Design review of the part built by this model. Coordinates are the model's own, in mm. Face numbers are marked on the shaded views. A direction names the side the tool comes from. Round coordinates to 2 decimals unless told otherwise and drop trailing zeros. Loops run counter-clockwise (first coordinate to the right, second up) from the corner with the lowest first, then second, coordinate; pieces in that order, holes last. Notation, with made-up numbers: (58, 52.25) -> (76, 52.25) arc R23 ccw to (76, 77.25) -> close; hole circle Ø2 at (37, 14). An arc over 180 degrees is marked (long way). Answer as CSV lines item,"result". Start each with the question number.
(1) For P1, Ø5, axis at y = -30.5, z = -21.5, coming from the -X side; P2, Ø13.5, axis at x = 10.37, z = 11.81, coming from the +Y side; P3, Ø15.5, axis at y = -61.5, z = -8.5, coming from the +X side; P4, Ø5, axis at y = -60.5, z = 20.5, coming from the +X side, all flat-tipped, find the tip position at first contact; note any pin that passes through.
(2) Take a section at B-B, the plane z = 25. State how many separate pieces and enclosed holes the cut face has, and give its area (3 significant figures).
(3) Take a section at D-D, the plane z = -8.5. Write out the cut boundary in (x, y), and give its area (3 significant figures).
(4) Draft analysis for pull direction X (two halves, no side actions). For the marked faces 5, 6, 7 and 8, state which applies: +X half, -X half, draft (parallel to the pull), parting line (faces both ways), or undercut.
(5) To check wall thickness, follow line 1 (Z direction, x = -20, y = -85.5); line 2 (Z direction, x = -42.5, y = -11); line 3 (X direction, y = -8, z = -27). State the ranges of each line that lie inside material, in increasing order. Write a range as from..to.
(6) Machinability: for the marked faces 1, 2, 3 and 4, which of the approach directions +Z, -Z, +X, -X, +Y, -Y give a long, thin tool a straight path to every point of the face, cutting with its end or side? Answer none if there is none.
(7) Take a section at C-C, the plane x = -11.5. Write out the cut boundary in (y, z).
(8) Take a section at A-A, the plane y = -42. Write out the cut boundary in (x, z).
from build123d import *

# Parameters (mm, degrees)
F1_DEPTH = 93.98
F2_R     = 6.626037
F2_R_2   = 6.777955
F3_DEPTH = 25.4
F5_DEPTH = 37.846
F6_R     = 7.438968
F7_DEPTH = 128.778


with BuildPart() as f1:
    # F0 (on Front) → F1 (new body)
    with BuildSketch(Plane.XZ):
        Polygon((-34.248885, 46.336725), (-59.863597, 46.336725), (-59.863597, 0), (-28.492769, 0), (-28.492769, -31.083023), (10.93662, -31.083023), (10.93662, 0), (30.219607, 0), (30.219607, 11.224424), (18.131761, 27.917158), (0, 27.917158), (0, 11.224424), (-24.175683, 11.224424), (-24.175683, 27.917158), (-34.248885, 27.917158), align=None)
    extrude(amount=F1_DEPTH)

    # F2 (on face) → F3 (cut)
    with BuildSketch(Plane(origin=(25.156285, 0, 18.216628), x_dir=(0, 1, 0), z_dir=(0.809942, 0, 0.58651))):
        with Locations((-67.734443, 0)):
            Circle(F2_R)
        with Locations((-22.558866, 0)):
            Circle(F2_R_2)
    extrude(amount=-F3_DEPTH, mode=Mode.SUBTRACT)

    # F4 (on face) → F5 (cut)
    with BuildSketch(Plane.XY.offset(46.336725)):
        with BuildLine():
            add(Edge.make_bspline(
                [(-49.610309, -46.578269), (-57.791175, -46.578269), (-53.700742, -62.50973), (-49.610309, -78.441191), (-45.519876, -62.50973), (-41.429444, -46.578269), (-49.610309, -46.578269)],
                knots=[0, 0, 0, 2.094395, 2.094395, 4.18879, 4.18879, 6.283185, 6.283185, 6.283185], degree=2, weights=[1, 0.5, 1, 0.5, 1, 0.5, 1]))
        make_face()
        with BuildLine():
            add(Edge.make_bspline(
                [(-49.610309, -11.490341), (-56.510654, -11.490341), (-53.060482, -27.570017), (-49.610309, -43.649692), (-46.160137, -27.570017), (-42.709965, -11.490341), (-49.610309, -11.490341)],
                knots=[0, 0, 0, 2.094395, 2.094395, 4.18879, 4.18879, 6.283185, 6.283185, 6.283185], degree=2, weights=[1, 0.5, 1, 0.5, 1, 0.5, 1]))
        make_face()
    extrude(amount=-F5_DEPTH, mode=Mode.SUBTRACT)

    # F6 (on face) → F7 (cut)
    with BuildSketch(Plane.XZ.offset(93.98)):
        with Locations((10.366299, 11.81201)):
            Circle(F6_R)
    extrude(amount=-F7_DEPTH, mode=Mode.SUBTRACT)


solid = f1.part
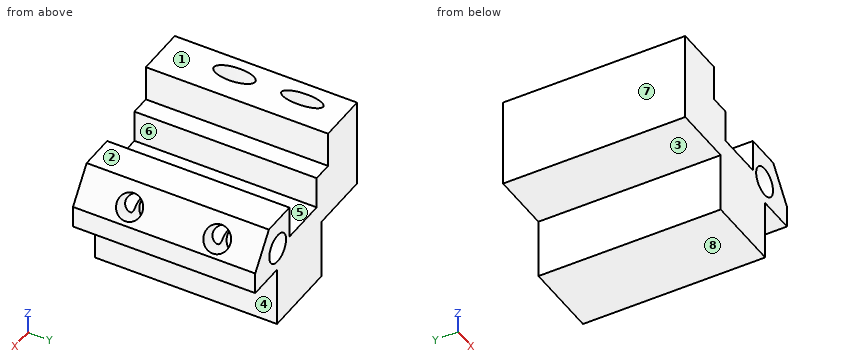
The answers:
1,P1,"x = -28.49"
1,P2,"through"
1,P3,"x = 10.94"
1,P4,"x = 25.31"
2,separate pieces,"2"
2,enclosed holes,"2"
2,area,"4,960 mm²"
3,outline,"(-28.49, -93.98) -> (10.94, -93.98) -> (10.94, 0) -> (-28.49, 0) -> close"
3,area,"3,710 mm²"
4,face 5,"undercut"
4,face 6,"undercut"
4,face 7,"-X half"
4,face 8,"draft"
5,line 1,"-31.08..11.22"
5,line 2,"0..46.34"
5,line 3,"-28.49..10.94"
6,face 1,"+Z, +X, -X, +Y, -Y"
6,face 2,"+Z, +X, +Y, -Y"
6,face 3,"-Z, -X, +Y, -Y"
6,face 4,"-Z, +X, +Y, -Y"
7,outline,"(-93.98, -31.08) -> (0, -31.08) -> (0, 11.22) -> (-93.98, 11.22) -> close"
8,outline,"(-59.86, 0) -> (-28.49, 0) -> (-28.49, -31.08) -> (10.94, -31.08) -> (10.94, 0) -> (30.22, 0) -> (30.22, 11.22) -> (18.13, 27.92) -> (0, 27.92) -> (0, 11.22) -> (-24.18, 11.22) -> (-24.18, 27.92) -> (-34.25, 27.92) -> (-34.25, 46.34) -> (-59.86, 46.34) -> close; hole circle Ø14.88 at (10.37, 11.81)"
